Source: CAD feature listing. Evaluate the final solid. Frame: model axes, mm. A direction names the side the tool comes from. Coordinates: 2 decimals unless noted, no trailing zeros. Order: outer loops, then holes, each group sorted by start corner. A loop starts at its lowest first (then second) coordinate and runs counter-clockwise, first axis right, second up.
```python
from build123d import *

# Parameters (mm, degrees)
F0_W     = 172
F0_H     = 172
F1_DEPTH = 10
F2_W     = 110
F2_H     = 110
F3_DEPTH = 45
F4_R     = 5


with BuildPart() as f1:
    # F0 (on Top) → F1 (new body)
    with BuildSketch(Plane.XY):
        Rectangle(F0_W, F0_H)
    extrude(amount=F1_DEPTH)

    # F2 (on Top) → F3 (cut)
    with BuildSketch(Plane.XY):
        Rectangle(F2_W, F2_H)
    extrude(amount=F3_DEPTH, mode=Mode.SUBTRACT)

    # F4
    f4_edges = [f1.edges().sort_by_distance(p)[0] for p in [
        (55, 55, 5),
        (55, -55, 5),
        (-55, -55, 5),
        (-55, 55, 5),
    ]]
    fillet(f4_edges, radius=F4_R)


solid = f1.part
```
1. Access query for faces 4 (the flat face through (-1, 86, 5)), 5 (the cylindrical face through (53, -54, 5)). Directions: +Z, -Z, +X, -X, +Y, -Y. A direction counts if a zero-diameter tool reaches every point of the face in a straight line with its end or side. Return the directions, or none.
2. Section query B-B, the plane x = -5. Output: boundary loops of the cut face in (y, z).
3. Draft query along Y for faces 1 (the flat face through (-55, -1, 5)), 2 (the flat face through (-1, -86, 5)), 3 (the flat face through (-1, 59, 10)). Return one class per face: +Y half, -Y half, draft (parallel to the pull), parting line (faces both ways), or undercut.
4. Section query A-A, the plane z = 6.75. Output: boundary loops of the cut face in (x, y).
5. Material intervals for line 1 along X through (y, z) = (-23.5, 1.25); line 2 along Y through (x, z) = (53, 9), sorted ascending.
Answer key:
1. face 4: +Z, -Z, +X, -X, +Y
1. face 5: +Z, -Z
2. outline: (-86, 0) - (-55, 0) - (-55, 10) - (-86, 10) - close; (55, 0) - (86, 0) - (86, 10) - (55, 10) - close
3. face 1: undercut
3. face 2: -Y half
3. face 3: draft
4. outline: (-86, -86) - (86, -86) - (86, 86) - (-86, 86) - close; hole (-55, -50) arc R5 ccw to (-50, -55) - (50, -55) arc R5 ccw to (55, -50) - (55, 50) arc R5 ccw to (50, 55) - (-50, 55) arc R5 ccw to (-55, 50) - close
5. line 1: x = -86 to -55, 55 to 86
5. line 2: y = -86 to -54, 54 to 86
